The model under review builds one solid part; all positions refer to its coordinate system, in mm. A direction names the side the tool comes from. Round coordinates to 2 decimals unless told otherwise and drop trailing zeros. Write each loop counter-clockwise with the first axis right and the second up, starting at its lowest first coordinate (ties: lowest second). Pieces come first, ordered by that corner, then holes. Notation, with made-up numbers: (-32, 26) -> (-12, 26) arc R20 cw to (-12, 50) -> close; hole circle Ø8 at (-22, -20.5). An arc over 180 degrees is marked (long way). Return JSON: item names as keys, results as strings. Group by question number.
1. Clearance check with flat-ended pins moving along their axes: P1, Ø4, axis at y = -20.5, z = 0, coming from the +X side; P2, Ø5.5, axis at x = 5, y = -30.5, coming from the -Z side; P3, Ø2.5, axis at x = 3.5, z = 20.5, coming from the +Y side. State where each tip first meets the part, or that it passes through.
2. Mouldability with a two-part tool opening along X and no side actions: class faces 1 (the cylindrical face through (9.57, -52.54, 22)), 2 (the flat face through (9, -50, 0)), 3 (the conical face through (0.38, -0.08, 20.3)) as pulls with the +X half, pulls with the -X half, needs draft (parallel to the pull), parting line crosses it, or undercut.
3. Tool access review of faces 4 (the cylindrical face through (3.465, -0.479, -19.345)), 5 (the cylindrical face through (3.465, -49.534, 16.357)), 6 (the cylindrical face through (3.465, -19.786, -12.227)), 7 (the cylindrical face through (8.96, -49.43, 7.4)): name each direction out of +Z, -Z, +X, -X, +Y, -Y from which nothing blocks a thin tool from reaching the whole face with its end or side.
4. For line 1 along Y through (x, z) = (3, 0); line 2 along Y through (x, z) = (4, 3); line 3 along Y through (x, z) = (9.75, 2.5), list the stretches that pass through material, from the lowest coordinate up. Write a range as from..to.
5. Take a section at A-A, the plane x = -1. Write out the cut boundary in (y, z), then the cut area to 3 significant figures.
6. Take a section at B-B, the plane x = 9.5. Give the number of separate pieces and of enclosed holes in the cut face, then the cut area to 3 significant figures.
from build123d import *

# Parameters (mm, degrees)
EXTRUDE_1_DEPTH        = 5
SKETCH_16_W            = 48
SKETCH_16_H            = 5
EXTRUDE_3_DEPTH        = 11
CUT_EXTRUDE_4_REACH    = 84.486
SKETCH_5_R             = 1.5
RIB_1_REACH            = 68.821
SKETCH_17_WALL_W       = 161.351231242
SKETCH_17_WALL_H       = 4
FILLET_1_R             = 2
HOLE_WIZARD_M3_2_D     = 2.5
HOLE_WIZARD_M3_2_DEPTH = 5
HOLE_WIZARD_M3_2_TIP   = 0.751075774
HOLE_WIZARD_M2_1_D     = 1.6
CHAMFER_1_SIZE         = 0.5
FILLET_2_R             = 10


with BuildPart() as part:
    # 草图3 → 旋转1 (revolve)
    with BuildSketch(Plane.XY, mode=Mode.PRIVATE) as revolve_1_sk:
        Polygon((6, 18), (-7, 18), (-7, 20), (0, 20), (0, 23), (6, 23), align=None)
    revolve(revolve_1_sk.sketch.rotate(Axis((-123.647082632, 0, 0), (1, 0, 0)), 90), axis=Axis((-123.647082632, 0, 0), (1, 0, 0)))

    # 草图4 → 凸台-拉伸1 (add)
    with BuildSketch(Plane(origin=(6, 0, 0), x_dir=(0, 0, -1), z_dir=(1, 0, 0))):
        with BuildLine():
            Line((-12, -19.62141687), (-12, -30))
            Line((-12, -30), (-16, -50))
            Line((-16, -50), (-24, -50))
            Line((-24, -50), (-24, -55))
            Line((-24, -55), (24, -55))
            Line((24, -55), (24, -50))
            Line((24, -50), (16, -50))
            Line((16, -50), (12, -30))
            Line((12, -30), (12, -19.62141687))
            ThreePointArc((12, -19.62141687), (9.092135156, -21.126596467), (6, -22.203603311))
            Line((6, -22.203603311), (6, -45))
            Line((6, -45), (-6, -45))
            Line((-6, -45), (-6, -22.203603311))
            ThreePointArc((-6, -22.203603311), (-9.092135156, -21.126596467), (-12, -19.62141687))
        make_face()
    extrude(amount=-EXTRUDE_1_DEPTH)

    # 草图16 → 凸台-拉伸3 (add)
    with BuildSketch(Plane(origin=(1, 0, 0), x_dir=(0, 0, -1), z_dir=(1, 0, 0))):
        with Locations((0, -52.5)):
            Rectangle(SKETCH_16_W, SKETCH_16_H)
    extrude(amount=EXTRUDE_3_DEPTH)

    # 草图5 → 切除-拉伸4 (cut, up to next)
    with BuildSketch(Plane.XZ.offset(55), mode=Mode.PRIVATE) as cut_extrude_4_sk1:
        with Locations(Location((9.5, 20.5, 0), (0, 0, 270))):
            Circle(SKETCH_5_R)
    cut_extrude_4_tool1 = extrude(cut_extrude_4_sk1.sketch, amount=-CUT_EXTRUDE_4_REACH, mode=Mode.PRIVATE) & part.part
    # 草图5 → 切除-拉伸4 (cut, up to next)
    with BuildSketch(Plane.XZ.offset(55), mode=Mode.PRIVATE) as cut_extrude_4_sk2:
        with Locations(Location((9.5, -20.5, 0), (0, 0, 270))):
            Circle(SKETCH_5_R)
    cut_extrude_4_tool2 = extrude(cut_extrude_4_sk2.sketch, amount=-CUT_EXTRUDE_4_REACH, mode=Mode.PRIVATE) & part.part
    # 草图5 → 切除-拉伸4 (cut, up to next)
    with BuildSketch(Plane.XZ.offset(55), mode=Mode.PRIVATE) as cut_extrude_4_sk3:
        with Locations(Location((3.5, -20.5, 0), (0, 0, 270))):
            Circle(SKETCH_5_R)
    cut_extrude_4_tool3 = extrude(cut_extrude_4_sk3.sketch, amount=-CUT_EXTRUDE_4_REACH, mode=Mode.PRIVATE) & part.part
    # 草图5 → 切除-拉伸4 (cut, up to next)
    with BuildSketch(Plane.XZ.offset(55), mode=Mode.PRIVATE) as cut_extrude_4_sk4:
        with Locations(Location((3.5, 20.5, 0), (0, 0, 270))):
            Circle(SKETCH_5_R)
    cut_extrude_4_tool4 = extrude(cut_extrude_4_sk4.sketch, amount=-CUT_EXTRUDE_4_REACH, mode=Mode.PRIVATE) & part.part
    add(cut_extrude_4_tool1.solids().sort_by_distance((9.5, -55, 20.5))[0], mode=Mode.SUBTRACT)
    add(cut_extrude_4_tool2.solids().sort_by_distance((9.5, -55, -20.5))[0], mode=Mode.SUBTRACT)
    add(cut_extrude_4_tool3.solids().sort_by_distance((3.5, -55, -20.5))[0], mode=Mode.SUBTRACT)
    add(cut_extrude_4_tool4.solids().sort_by_distance((3.5, -55, 20.5))[0], mode=Mode.SUBTRACT)

    # 草图17 wall → 筋1 (add, up to next)
    with BuildSketch(Plane(origin=(9, -37.5, 12), x_dir=(0.233372952475, -0.972387301981, 0), z_dir=(0.972387301981, 0.233372952475, 0)), mode=Mode.PRIVATE) as rib_1_sk1:
        with Locations((0, 2)):
            Rectangle(SKETCH_17_WALL_W, SKETCH_17_WALL_H)
    rib_1_tool1 = extrude(rib_1_sk1.sketch, amount=-RIB_1_REACH, mode=Mode.PRIVATE) - part.part
    rib_1 = rib_1_tool1.solids().sort_by_distance((9, -37.5, 12))[0]
    add(rib_1)

    # 镜向1: 筋1 across plane
    add(rib_1.mirror(Plane.XY))

    # 圆角1
    fillet_1_edges = [part.edges().sort_by_distance(p)[0] for p in [
        (9, -50, 12),
        (9, -50, 8),
        (9, -50, -8),
        (9, -50, -12),
        (3.5, -22.203603311, -6),
        (3.5, -19.62141687, -12),
        (3.5, -50, -16),
        (6.5, -50, -24),
        (6.5, -50, 24),
        (3.5, -50, 16),
        (3.5, -19.62141687, 12),
        (3.5, -22.203603311, 6),
        (3.5, -45, 6),
        (3.5, -45, -6),
    ]]
    fillet(fillet_1_edges, radius=FILLET_1_R - 0.0001)  # a hair under: the kernel refuses the full size

    # M3 螺纹孔2
    with Locations(Plane(origin=(6, 0, 0), x_dir=(0, 0, -1), z_dir=(1, 0, 0))):
        with Locations((0, 20.5), (-20.5, 0), (0, -20.5), (20.5, 0)):
            Hole(HOLE_WIZARD_M3_2_D / 2, depth=HOLE_WIZARD_M3_2_DEPTH)
            with Locations((0, 0, -(HOLE_WIZARD_M3_2_DEPTH + HOLE_WIZARD_M3_2_TIP / 2))):  # 118° drill point
                Cone(0, HOLE_WIZARD_M3_2_D / 2, HOLE_WIZARD_M3_2_TIP, mode=Mode.SUBTRACT)

    # M2 螺纹孔1 (through all)
    with Locations(Plane(origin=(6, 0, 0), x_dir=(0, 0, -1), z_dir=(1, 0, 0))):
        with Locations((-15.202795796, 15.202795796), (15.202795796, 15.202795796), (15.202795796, -15.202795796), (-15.202795796, -15.202795796)):
            Hole(HOLE_WIZARD_M2_1_D / 2)

    # 倒角1
    chamfer_1_edges = [part.edges().sort_by_distance(p)[0] for p in [
        (6, 0, -18),
        (-7, 0, -20),
    ]]
    chamfer(chamfer_1_edges, length=CHAMFER_1_SIZE)

    # 圆角2
    fillet_2_edges = [part.edges().sort_by_distance(p)[0] for p in [
        (3.5, -30, 12),
        (3.5, -30, -12),
    ]]
    fillet(fillet_2_edges, radius=FILLET_2_R)


solid = part.part
Output:
{
 "1": {"P1": "stops at x = 6", "P2": "stops at z = -12.65", "P3": "stops at y = 12.59"},
 "2": {"face 1": "undercut", "face 2": "needs draft", "face 3": "pulls with the +X half"},
 "3": {"face 4": "+X", "face 5": "+Z, +X, -X", "face 6": "-Z, +X, -X", "face 7": "+X, +Y"},
 "4": {"line 1": "y = -55..-45, -23..-21.75, -19.25..-18, 18..19.25, 21.75..23", "line 2": "y = -55..-45, -22.8..-17.75, 17.75..22.8", "line 3": "y = -55..-50"},
 "5": {"outline": "circle Ø40 at (0, 0); hole circle Ø36 at (0, 0)", "area": "239 mm^2"},
 "6": {"separate pieces": "3", "enclosed holes": "0", "area": "295 mm^2"}
}
